```python
from build123d import *

# Parameters (mm, degrees)
MAIN_BASE_DIM_W                            = 73.60000012
MAIN_BASE_DIM_H                            = 74.750000106
MAIN_BASE_DEPTH                            = 2.54
CSK_FOR_10_FLAT_HEAD_MACHINE_SCREW_2_COUNT = 2
CSK_FOR_10_FLAT_HEAD_MACHINE_SCREW_2_PITCH = 40.130936127
CSK_FOR_10_FLAT_HEAD_MACHINE_SCREW_3_COUNT = 2
CSK_FOR_10_FLAT_HEAD_MACHINE_SCREW_3_PITCH = 54.55000006
CSK_FOR_10_FLAT_HEAD_MACHINE_SCREW_4_COUNT = 2
CSK_FOR_10_FLAT_HEAD_MACHINE_SCREW_4_PITCH = 40.130936127
CONER_CUT_DEPTH                            = 2.54
F_1IN_FILLET_R                             = 2.54


with BuildPart() as part:
    # Main_Base_Dim → Main_Base (new body)
    with BuildSketch(Plane(origin=(0, 0, 0), x_dir=(1, 0, 0), z_dir=(0, 1, 0))):
        with Locations((36.80000006, 37.375000053)):
            Rectangle(MAIN_BASE_DIM_W, MAIN_BASE_DIM_H)
    extrude(amount=MAIN_BASE_DEPTH)

    # Sketch4 → CSK for #10 Flat Head Machine Screw (100)1 (revolve, cut)
    with BuildSketch(Plane(origin=(9.52500003, 2.54, -37.375000053), x_dir=(0, 0, 1), z_dir=(1, 0, 0))):
        Polygon((0, 0), (0, 2.54), (2.5527, 2.54), (2.5527, 1.960808018), (4.8895, 0), align=None)
    csk_for_10_flat_head_machine_screw_100 = revolve(axis=Axis((9.52500003, 8.89, -37.375000053), (0, -1, 0)), mode=Mode.SUBTRACT)

    # CSK for _10 Flat Head Machine Screw  2: CSK for #10 Flat Head Machine Screw (100)1 ×2
    with Locations(*[Vector(0.679650232, 0, 0.73353634) * (i * CSK_FOR_10_FLAT_HEAD_MACHINE_SCREW_2_PITCH) for i in range(1, CSK_FOR_10_FLAT_HEAD_MACHINE_SCREW_2_COUNT)]):
        add(csk_for_10_flat_head_machine_screw_100, mode=Mode.SUBTRACT)

    # CSK for _10 Flat Head Machine Screw  3: CSK for #10 Flat Head Machine Screw (100)1 ×2
    with Locations(*[(i * CSK_FOR_10_FLAT_HEAD_MACHINE_SCREW_3_PITCH, 0, 0) for i in range(1, CSK_FOR_10_FLAT_HEAD_MACHINE_SCREW_3_COUNT)]):
        add(csk_for_10_flat_head_machine_screw_100, mode=Mode.SUBTRACT)

    # CSK for _10 Flat Head Machine Screw  4: CSK for #10 Flat Head Machine Screw (100)1 ×2
    with Locations(*[Vector(0.679650232, 0, -0.73353634) * (i * CSK_FOR_10_FLAT_HEAD_MACHINE_SCREW_4_PITCH) for i in range(1, CSK_FOR_10_FLAT_HEAD_MACHINE_SCREW_4_COUNT)]):
        add(csk_for_10_flat_head_machine_screw_100, mode=Mode.SUBTRACT)

    # Corner_Cut_Dim → Coner_Cut (cut)
    with BuildSketch(Plane(origin=(0, 2.54, 0), x_dir=(1, 0, 0), z_dir=(0, 1, 0))):
        Polygon((0, 0), (0, 19.05), (19.05, 0), align=None)
        Polygon((54.55000012, 0), (73.60000012, 0), (73.60000012, 19.05), align=None)
        Polygon((73.60000012, 74.750000106), (73.60000012, 55.700000106), (54.55000012, 74.750000106), align=None)
        Polygon((0, 55.700000106), (19.05, 74.750000106), (0, 74.750000106), align=None)
    extrude(amount=-CONER_CUT_DEPTH, mode=Mode.SUBTRACT)

    # .1in_Fillet
    f_1in_fillet_edges = [part.edges().sort_by_distance(p)[0] for p in [
        (19.05, 1.27, -74.750000106),
        (0, 1.27, -55.700000106),
        (73.60000012, 1.27, -55.700000106),
        (54.55000012, 1.27, -74.750000106),
        (73.60000012, 1.27, -19.05),
        (54.55000012, 1.27, 0),
        (0, 1.27, -19.05),
        (19.05, 1.27, 0),
    ]]
    fillet(f_1in_fillet_edges, radius=F_1IN_FILLET_R)


solid = part.part
```
The model under review builds one solid part; all positions refer to its coordinate system, in mm. Coordinates: 2 decimals unless noted, no trailing zeros. Write each loop counter-clockwise with the first axis right and the second up, starting at its lowest first coordinate (ties: lowest second). Pieces come first, ordered by that corner, then holes.
1) To check wall thickness, follow probe 1 along Z at (x, y) = (16, 1.2); probe 2 along Z at (x, y) = (66, 1.9); probe 3 along Z at (x, y) = (7, 1.8). State the ranges of each line that lie inside material, in increasing order.
2) We need section D-D on z = -16.5. State the section outline as (x, y) points.
3) We need section B-B on y = 1.85. Count the separate pieces of the cut face and the enclosed holes in it, then the cut area to 3 significant figures.
4) The part is to be moulded in two halves that separate along Z. For faces 1 (the face through (64.2, 1.3, -65.1)), 2 (the face through (36, 0, -38)), 3 (the face through (37.834, 0.702, -5.444)), say which applies: pulls with the +Z half, pulls with the -Z half, needs draft (parallel to the pull), parting line crosses it, or undercut.
5) Clearance check with flat-ended pins moving along their axes: pin 1 Ø6.5 at (x, z) = (9.525, -37.375) entering from +Y; pin 2 Ø1 at (y, z) = (1, -18) entering from -X; pin 3 Ø1 at (x, z) = (34.5, -67) entering from -Y. State where each tip first meets the part, or that it passes through.
6) We need section C-C on x = 56.5. State the section outline as (y, z) points.
7) We need section A-A on x = 36.8. State the section outline as (y, z) points.
Answer list:
1. probe 1: z = -71.7 to -3.05
1. probe 2: z = -63.3 to -41.03, -33.72 to -11.45
1. probe 3: z = -62.7 to -40.49, -34.26 to -12.05
2. outline: (2.55, 0) - (71.05, 0) - (71.05, 2.54) - (2.55, 2.54) - close
3. separate pieces: 1
3. enclosed holes: 4
3. area: 4,570 mm2
4. face 1: pulls with the -Z half
4. face 2: needs draft
4. face 3: undercut
5. pin 1: stops at y = 1.16
5. pin 2: stops at x = 0.57
5. pin 3: stops at y = 0
6. outline: (0, -72.8) - (2.54, -72.8) - (2.54, -1.95) - (0, -1.95) - close
7. outline: (0, -74.75) - (2.54, -74.75) - (2.54, -71.7) - (0.58, -69.37) - (0, -69.37) - close; (0, -64.26) - (0.58, -64.26) - (2.54, -61.92) - (2.54, -12.83) - (0.58, -10.49) - (0, -10.49) - close; (0, -5.38) - (0.58, -5.38) - (2.54, -3.05) - (2.54, 0) - (0, 0) - close
